The listing builds one solid part. Answer for the finished solid, in the listing's coordinates (mm). A direction names the side the tool comes from. Give positions to 0.01 mm unless a question says otherwise; leave off trailing zeros. Order: outer loops, then holes, each group sorted by start corner. A loop starts at its lowest first (then second) coordinate and runs counter-clockwise, first axis right, second up.
```python
from build123d import *

# Parameters (mm, degrees)
BOSS_EXTRU_1_DEPTH      = 220
ENL_V_MAT_EXTRU_1_REACH = 222
ESQUISSE4_W             = 200
ESQUISSE4_H             = 250
ENL_V_MAT_EXTRU_2_DEPTH = 200
ESQUISSE5_W             = 220
ESQUISSE5_H             = 30
BOSS_EXTRU_2_DEPTH      = 2
ESQUISSE7_W             = 220
ESQUISSE7_H             = 2
BOSS_EXTRU_4_DEPTH      = 100
ESQUISSE8_W             = 2
ESQUISSE8_H             = 28
BOSS_EXTRU_5_DEPTH      = 100


with BuildPart() as part:
    # Esquisse1 → Boss.-Extru.1 (new body)
    with BuildSketch(Plane(origin=(0, 0, 0), x_dir=(0, 0, -1), z_dir=(1, 0, 0))):
        with BuildLine():
            Line((0, 0), (0, -250))
            ThreePointArc((0, -250), (5, -255), (10, -250))
            Line((10, -250), (10, 0))
            ThreePointArc((10, 0), (5, 5), (0, 0))
        make_face()
    extrude(amount=BOSS_EXTRU_1_DEPTH)

    # Esquisse2 → Enlèv. mat.-Extru.1 (cut, up to next)
    with BuildSketch(Plane.ZY, mode=Mode.PRIVATE) as enl_v_mat_extru_1_sk1:
        with BuildLine():
            Line((-7.5, 0), (-7.5, -250))
            ThreePointArc((-7.5, -250), (-5, -252.5), (-2.5, -250))
            Line((-2.5, -250), (-2.5, 0))
            ThreePointArc((-2.5, 0), (-5, 2.5), (-7.5, 0))
        make_face()
    enl_v_mat_extru_1_tool1 = extrude(enl_v_mat_extru_1_sk1.sketch, amount=-ENL_V_MAT_EXTRU_1_REACH, mode=Mode.PRIVATE) & part.part
    add(enl_v_mat_extru_1_tool1.solids().sort_by_distance((0, -125, -5))[0], mode=Mode.SUBTRACT)

    # Esquisse4 → Enlèv. mat.-Extru.2 (cut)
    with BuildSketch(Plane.XY):
        with Locations((110, -125)):
            Rectangle(ESQUISSE4_W, ESQUISSE4_H)
    extrude(amount=-ENL_V_MAT_EXTRU_2_DEPTH, mode=Mode.SUBTRACT)

    # Esquisse5 → Boss.-Extru.2 (add)
    with BuildSketch(Plane.XY):
        with Locations((110, -155)):
            Rectangle(ESQUISSE5_W, ESQUISSE5_H)
    extrude(amount=BOSS_EXTRU_2_DEPTH)

    # Esquisse7 → Boss.-Extru.4 (add)
    with BuildSketch(Plane.XY.offset(2)):
        with Locations((110, -169)):
            Rectangle(ESQUISSE7_W, ESQUISSE7_H)
    extrude(amount=BOSS_EXTRU_4_DEPTH)

    # Esquisse8 → Boss.-Extru.5 (add)
    with BuildSketch(Plane.XY.offset(2)):
        with Locations((1, -154)):
            Rectangle(ESQUISSE8_W, ESQUISSE8_H)
        with Locations((219, -154)):
            Rectangle(ESQUISSE8_W, ESQUISSE8_H)
    extrude(amount=BOSS_EXTRU_5_DEPTH)


solid = part.part
```
1) Find section C-C (z = 8). Write down the section's boundary in (x, y).
Geometry says:
outline: (0, -170) - (220, -170) - (220, -140) - (218, -140) - (218, -168) - (2, -168) - (2, -140) - (0, -140) - close
2) Find section B-B (y = -106). Write down the section's boundary in (x, z).
Geometry says:
outline: (0, -10) - (10, -10) - (10, -7.5) - (0, -7.5) - close; (0, -2.5) - (10, -2.5) - (10, 0) - (0, 0) - close; (210, -10) - (220, -10) - (220, -7.5) - (210, -7.5) - close; (210, -2.5) - (220, -2.5) - (220, 0) - (210, 0) - close
3) Given P1, Ø3, axis at x = 216, y = -215.5, coming from the +Z side; P2, Ø10, axis at x = 197.5, y = -160, coming from the -Z side; P3, Ø0.8, axis at x = 126.5, z = -2, coming from the +Y side; P4, Ø0.8, axis at y = -105.5, z = -1.5, coming from the -X side, each flat-ended and moving along its own axis, determine where each tip first touches the part or whether it passes through.
Geometry says:
P1: stops at z = 0
P2: stops at z = 0
P3: stops at y = 4.27
P4: stops at x = 0
4) For a pull along X with two mould halves and no side action, classify faces 1 (the flat face through (0, -145, 37)), 2 (the flat face through (109, -155, 0)), 3 (the flat face through (5, -127, -10)) as +X half, -X half, draft (parallel to the pull), parting line (faces both ways), or undercut.
Geometry says:
face 1: -X half
face 2: undercut
face 3: draft
5) A tool of negligible diameter and unlimited length cuts with its end or side. For faces 4 (the flat face through (220, -145, 37)), 5 (the flat face through (5, -209, 0)), 6 (the flat face through (5, -69, 0)), 7 (the flat face through (108, -154, 2)), 8 (the flat face through (215, -123, -7.5)), from which of +Z, -Z, +X, -X, +Y, -Y can it reach the whole face along a straight path? Write none if from no direction.
Geometry says:
face 4: +Z, -Z, +X, +Y, -Y
face 5: +Z, +X, -X, -Y
face 6: +Z, +X, -X, +Y
face 7: +Z, +Y
face 8: +X, -X
6) Find section A-A (x = 31). Write down the section's boundary in (y, z).
Geometry says:
outline: (-250, -10) - (-250, -7.5) arc R2.5 cw to (-250, -2.5) - (-250, 0) arc R5 ccw to start; (-170, 0) - (-140, 0) - (-140, 2) - (-168, 2) - (-168, 102) - (-170, 102) - close; (0, -10) arc R5 ccw to (0, 0) - (0, -2.5) arc R2.5 cw to (0, -7.5) - close
7) Straight lines are drawn through the part: probe 1 along Y at (x, z) = (149.5, -5); probe 2 along Y at (x, z) = (164.5, 28.5); probe 3 along Z at (x, y) = (53, -165). For each, find the intervals that lie inside material, in ascending order.
Geometry says:
probe 1: y = -255 to -252.5, 2.5 to 5
probe 2: y = -170 to -168
probe 3: z = 0 to 2
